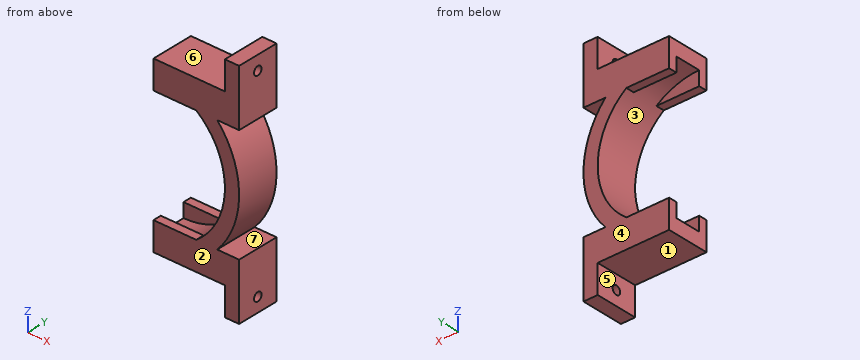
Autodesk Inventor part; units mm, degrees
ref_plane "YZ Plane" through (0, 0, 0) normal (1, 0, 0) x (0, 1, 0)
ref_plane "XZ Plane" through (0, 0, 0) normal (0, 1, 0) x (-1, 0, 0)
ref_plane "XY Plane" through (0, 0, 0) normal (0, 0, 1) x (1, 0, 0)
sketch "Boceto1" plane through (0, 0, 0) normal (0, 1, 0) x (-1, 0, 0)
  arc A0 (0, 25.125) -> (0, -25.125) centre (0, 0) ccw
  arc A1 (0, 30.125) -> (0, -30.125) centre (0, 0) ccw
  line L0 (0, 30.125) -> (-30.125, 30.125)
  line L1 (-30.125, 30.125) -> (-30.125, 20.125)
  line L2 (-30.125, 20.125) -> (-22.4165, 20.125)
  line L3 (6.35, 0) -> (-9.525, 0)
  line L4 (0, -30.125) -> (-30.125, -30.125)
  line L5 (-30.125, -30.125) -> (-30.125, -20.125)
  line L6 (-30.125, -20.125) -> (-22.4165, -20.125)
  line L7 (0, 30.125) -> (0, 25.125)
  line L8 (0, -25.125) -> (0, -30.125)
  dimension "d0" = 50.25
  dimension "d1" = 5
  dimension "d2" = 10
extrude "Extrusión1" add sketch "Boceto1" along normal blind 15
sketch "Boceto2" plane through (0, 15, 0) normal (0, 1, 0) x (1, 0, 0)
  arc A0 (0, -25.125) -> (0, 25.125) centre (0, 0) ccw
  line L0 (0, 25.125) -> (0, 20.125)
  line L1 (0, 20.125) -> (15.0416, 20.125)
  dimension "d5" = 5
extrude "Extrusión2" add sketch "Boceto2" against normal blind 2.95
mirror "Simetría1" about plane through (0, 0, 0) normal (0, 0, 1) of "Extrusión2"
sketch "Boceto3" plane through (0, 0, 0) normal (0, -1, 0) x (1, 0, 0)
  arc A0 (0, -25.125) -> (15.0416, -20.125) centre (0, 0) ccw
  line L0 (0, -20.125) -> (0, -25.125)
  line L1 (0, -25.125) -> (0, -20.125)
  line L2 (0, -20.125) -> (15.0416, -20.125)
extrude "Extrusión3" add sketch "Boceto3" against normal blind 2.95
mirror "Simetría2" about plane through (0, 0, 0) normal (0, 0, 1) of "Extrusión3"
sketch "Boceto4" plane through (0, 0, 30.125) normal (0, 0, 1) x (1, 0, 0)
  line L0 (30.125, 0) -> (30.125, 15)
  line L1 (30.125, 15) -> (25.125, 15)
  line L2 (25.125, 15) -> (25.125, 0)
  line L3 (25.125, 0) -> (30.125, 0)
  line L4 (30.125, 0) -> (30.125, 15)
  point P0 (0, 0)
  dimension "d10" = 5
extrude "Extrusión4" add sketch "Boceto4" along normal blind 10
sketch "Boceto5" plane through (25.125, 0, 30.125) normal (-1, 0, 0) x (0, 0, 1)
  line L0 (-10, 15) -> (10, 15)
  line L1 (-10, 0) -> (0, 0)
  line L2 (10, 15) -> (0, 15)
  line L3 (0, 15) -> (0, 0)
  line L4 (0, 0) -> (10, 0)
  line L5 (10, 0) -> (10, 15)
  circle A0 centre (5, 7.5) radius 1.5
  point P0 (-30.125, 0)
  dimension "d13" = 3
extrude "Extrusión5" cut sketch "Boceto5" against normal blind 10 contours A0
mirror "Simetría3" about plane through (0, 0, 0) normal (0, 0, 1) of "Extrusión4", "Extrusión5"
properties part number "LensSupport" material "Plástico ABS"
Read the model definition and answer for the solid it produces. Units are mm, in the model's axes. Face numbers are marked on the shaded views. A direction names the side the tool comes from. Give positions to 0.01 mm unless a question says otherwise; leave off trailing zeros. Write each loop counter-clockwise with the first axis right and the second up, starting at its lowest first coordinate (ties: lowest second). Pieces come first, ordered by that corner, then holes. Notation, with made-up numbers: M 86,35.25 L 136,35.25 A24 ccw 136,55.25 Z; hole C -19.5,29 d6. An arc over 180 degrees is marked long. One line per item, written item: value. Start each with the question number.
(1) Determine the mould class of the marked faces 1, 2 and 3 for opening direction Z: pulls with the +Z half, pulls with the -Z half, needs draft (parallel to the pull), parting line crosses it, or undercut.
(2) Flat-ended cylindrical pins translate along their axes: pin 1 Ø4.5 at (x, y) = (13, 8) entering from -Z (3 decimals); pin 2 Ø4 at (y, z) = (7.5, 35.125) entering from -X (3 decimals); pin 3 Ø0.9 at (x, y) = (6, 1.5) entering from +Z (3 decimals); pin 4 Ø2.5 at (y, z) = (7.5, -35.125) entering from -X. Find the tip coordinate at first contact, or state that the pin passes through.
(3) Find section C-C (x = 7). Determine the outline of the cut face in (y, z) (3 decimals).
(4) Find section B-B (x = 26). Determine the outline of the cut face in (y, z) (3 decimals).
(5) Find the intervals of material crossed by line 1 (Z direction, x = 3.5, y = 2.5) (3 decimals); line 2 (Y direction, x = 6, z = 23.5); line 3 (Z direction, x = 3, y = 8.75) (3 decimals), in increasing order.
(6) Find section A-A (y = 7.5). Give the number of separate pieces and of enclosed holes in the cut face, plus the area to 3 significant figures.
(7) A tool of negligible diameter and unlimited length cuts with its end or side. For the marked faces 4, 5, 6 and 7, from which of +Z, -Z, +X, -X, +Y, -Y can it reach the whole face along a straight path? Write none if from no direction.
Results below:
1. face 1: pulls with the -Z half
1. face 2: needs draft
1. face 3: undercut
2. pin 1: stops at z = -30.125
2. pin 2: stops at x = 25.125
2. pin 3: stops at z = 30.125
2. pin 4: passes through
3. outline: M 0,-30.125 L 15,-30.125 L 15,-20.125 L 12.05,-20.125 L 12.05,-24.13 L 2.95,-24.13 L 2.95,-20.125 L 0,-20.125 Z; M 0,20.125 L 2.95,20.125 L 2.95,24.13 L 12.05,24.13 L 12.05,20.125 L 15,20.125 L 15,30.125 L 0,30.125 Z
4. outline: M 0,-40.125 L 15,-40.125 L 15,-20.125 L 0,-20.125 Z; M 0,-15.216 L 15,-15.216 L 15,15.216 L 0,15.216 Z; M 0,20.125 L 15,20.125 L 15,40.125 L 0,40.125 Z; hole C 7.5,-35.125 d3; hole C 7.5,35.125 d3
5. line 1: z = -30.125 to -20.125, 20.125 to 30.125
5. line 2: y = 0 to 2.95, 12.05 to 15
5. line 3: z = -30.125 to -24.945, 24.945 to 30.125
6. separate pieces: 3
6. enclosed holes: 0
6. area: 796 mm^2
7. face 4: +Z, -Z, +X, -X, +Y
7. face 5: -Z, -X, +Y, -Y
7. face 6: +Z, -X, +Y, -Y
7. face 7: +X, +Y, -Y
